from build123d import *

# Parameters (mm, degrees)
F3_D     = 5.1054
F3_DEPTH = 22.225
F3_TIP   = 1.5338169022
F4_R     = 0.762
F5_R     = 0.254
F6_W     = 47.0435560763
F6_H     = 4.7625


with BuildPart() as f1:
    # F0 (on Right) → F1 (revolve)
    with BuildSketch(Plane.YZ):
        Polygon((-24.13, 0), (25.4, 0), (25.4, 9.525), (0, 9.525), (0, 6.096), (-24.13, 5.4941811878), align=None)
    revolve(axis=Axis((0, 0.635, 0), (0, 1, 0)))

    # F3
    with Locations(Plane.XZ.offset(24.13)):
        with Locations((0, 0)):
            Hole(F3_D / 2, depth=F3_DEPTH)
            with Locations((0, 0, -(F3_DEPTH + F3_TIP / 2))):  # 118° drill point
                Cone(0, F3_D / 2, F3_TIP, mode=Mode.SUBTRACT)

    # F4
    f4_edges = [f1.edges().sort_by_distance(p)[0] for p in [
        (0, 0, -6.096),
    ]]
    fillet(f4_edges, radius=F4_R)

    # F5
    f5_edges = [f1.edges().sort_by_distance(p)[0] for p in [
        (0, 0, -9.525),
        (0, 25.4, -9.525),
        (0, -24.13, -5.494181),
    ]]
    fillet(f5_edges, radius=F5_R)

    # F6 (on Right) → F7 (revolve, cut)
    with BuildSketch(Plane.YZ):
        with Locations((26.6967780381, 2.38125)):
            Rectangle(F6_W, F6_H)
    revolve(axis=Axis((0, 26.6967780381, 0), (0, -1, 0)), mode=Mode.SUBTRACT)


solid = f1.part
Can you work these out from the model? Positions are in its coordinate system, mm. A direction names the side the tool comes from. Round coordinates to 2 decimals unless told otherwise and drop trailing zeros. Write each loop counter-clockwise with the first axis right and the second up, starting at its lowest first coordinate (ties: lowest second). Pieces come first, ordered by that corner, then holes. Notation, with made-up numbers: M 15,86.25 L 43,86.25 A16 cw 43,90.25 Z; hole C -35,31 d2. An arc over 180 degrees is marked long. Use CSV: the item, a comma, the result in double quotes.
(1) Imagine slicing it at B-B (y = -11.5). Write out the boundary of the cut face in (x, z), plus the area to 3 significant figures.
Check values:
outline,"C 0,0 d11.62; hole C 0,0 d5.11"
area,"85.5 mm^2"
(2) On a 3-axis mill with a long thin cutter (end or side, diameter ignored), from which of +Z, -Z, +X, -X, +Y, -Y can I reach the whole of each face in a straight line? I mean faces 4 (the flat face through (-4, 25.4, -4)), 5 (the flat face through (0, 3.175, 0)), 6 (the cylindrical face through (-2.435, -12.862, 0.767)). Say none if no direction works.
Check values:
face 4,"+Z, -Z, +X, -X, +Y"
face 5,"+Y"
face 6,"-Y"
(3) I need wall thicknesses on line 1 along X through (y, z) = (12.5, 0) (1 decimal); line 2 along X through (y, z) = (-16, 1.5); line 3 along Z through (x, y) = (0, -17.5). Which ranges of each line are inside material? Lowest first, please.
Check values:
line 1,"-9.5 to -4.8, 4.8 to 9.5"
line 2,"-5.5 to -2.07, 2.07 to 5.5"
line 3,"-5.66 to -2.55, 2.55 to 5.66"
(4) We'd pull the mould along Z, two halves only. Please class faces 1 (the flat face through (-7, 0, -1)), 2 (the cylindrical face through (2.9, 14.44, -3.78)), 3 (the cylindrical face through (-5.796, 12.526, -7.559)): +Z half, -Z half, draft (parallel to the pull), parting line (faces both ways), or undercut.
Check values:
face 1,"draft"
face 2,"undercut"
face 3,"parting line"
(5) I'm going to push flat-ended pins straight in: pin 1 (6 mm diameter, centred on x = 2, y = -16.5, fed in from +Z); pin 2 (3 mm diameter, centred on x = 0.5, z = 3, fed in from +Y) (3 decimals); pin 3 (5.5 mm diameter, centred on x = -1, z = -1.5, fed in from -Y); pin 4 (8 mm diameter, centred on x = 6.5, y = -14.5, fed in from -Z). Where does each tip first touch, or does it pass through?
Check values:
pin 1,"z = 5.74"
pin 2,"y = 3.175"
pin 3,"y = -24.13"
pin 4,"z = -5.16"
